Autodesk Inventor part; units mm, degrees
ref_plane "YZ Plane" through (0, 0, 0) normal (1, 0, 0) x (0, 1, 0)
ref_plane "XZ Plane" through (0, 0, 0) normal (0, 1, 0) x (-1, 0, 0)
ref_plane "XY Plane" through (0, 0, 0) normal (0, 0, 1) x (1, 0, 0)
sketch "Sketch1" plane through (0, 0, 0) normal (0, 1, 0) x (-1, 0, 0)
  line L0 (0, 0) -> (0, -57.15)
  line L1 (0, -57.15) -> (31.75, -57.15)
  line L2 (31.75, -57.15) -> (31.75, -82.55)
  line L3 (31.75, -82.55) -> (-57.15, -82.55)
  line L4 (-57.15, -82.55) -> (-57.15, -57.15)
  line L5 (-57.15, -57.15) -> (-25.4, -57.15)
  line L6 (-25.4, -57.15) -> (-25.4, 0)
  line L7 (-25.4, 0) -> (0, 0)
  dimension "d0" = 88.9
  dimension "d1" = 25.4
  dimension "d2" = 25.4
  dimension "d3" = 31.75
  dimension "d4" = 82.55
extrude "Extrusion1" add sketch "Sketch1" along normal blind 2.286
fillet "Fillet1" radius 3.175 2 edges at (25.4, 1.143, -57.15) (0, 1.143, -57.15)
chamfer "Chamfer1" distance 1.5875 angle 45 6 edges at (0, 1.143, 0) (25.4, 1.143, 0) (57.15, 1.143, -57.15) (57.15, 1.143, -82.55) (-31.75, 1.143, -57.15) (-31.75, 1.143, -82.55)
sketch "Sketch2" plane through (0, 2.286, 0) normal (0, 1, 0) x (1, 0, 0)
  line L0 (55.5625, 82.55) -> (-30.1625, 82.55)
  line L1 (25.4, 1.5875) -> (25.4, 53.975)
  point P0 (0, 0)
  point P1 (12.7, 69.85)
  dimension "d11" = 12.7
  dimension "d12" = 12.7
hole "Hole1" at (12.7, 2.286, -69.85) direction (0, -1, 0) diameter 4.1402 end through all
pattern_linear "Rectangular Pattern1" count 6 spacing 12.7 along (0, 0, 1) of "Hole1"
pattern_linear "Rectangular Pattern2" count 7 spacing 12.7 along (-1, 0, 0) of "Hole1" first direction both ways yes
properties part number "T Gusset"
Source: CAD feature listing. Evaluate the final solid. Frame: model axes, mm. A direction names the side the tool comes from. Coordinates: 2 decimals unless noted, no trailing zeros. Loops run counter-clockwise (first coordinate to the right, second up) from the corner with the lowest first, then second, coordinate; pieces in that order, holes last. Notation, with made-up numbers: (44.5, 31.5) - (102.5, 31.5) arc R24 ccw to (102.5, 52.5) - close; hole circle Ø1 at (-39, 68). An arc over 180 degrees is marked (long way). Return JSON: item names as keys, results as strings.
Q1. Material intervals for line 1 along Z through (x, y) = (-12.5, 0.7); line 2 along X through (y, z) = (1.3, -9); line 3 along X through (y, z) = (0.7, -44.45), sorted ascending.
Results:
{"line 1": "-82.55 to -71.91, -67.79 to -57.15", "line 2": "0 to 25.4", "line 3": "0 to 10.63, 14.77 to 25.4"}
Q2. Section B-B, the plane x = -25.4. Return loops of the section in (y, z), plus the area to 3 significant figures.
Results:
{"outline": "(0, -82.55) - (2.29, -82.55) - (2.29, -71.92) - (0, -71.92) - close; (0, -67.78) - (2.29, -67.78) - (2.29, -57.15) - (0, -57.15) - close", "area": "48.6 mm2"}
Q3. Mould query, pull axis Z, two halves, no side actions, for faces 3 (the cylindrical face through (38.01, 1.13, -71.92)), 4 (the flat face through (57.15, 1, -70)), 5 (the flat face through (13, 1, 0)). Classes: released by +Z, released by -Z, zero draft, split by the parting line, or undercut.
Results:
{"face 3": "undercut", "face 4": "zero draft", "face 5": "released by +Z"}
Q4. Contact query for flat-ended pins moving along their axis: P1, Ø1.1, axis at y = 1, z = -28, coming from the +X side; P2, Ø3.5, axis at x = 0, z = -69.85, coming from the -Y side; P3, Ø0.7, axis at x = 46.5, y = 1, coming from the +Z side. Output: stop coordinate, or through.
Results:
{"P1": "x = 25.4", "P2": "through", "P3": "z = -57.15"}
Q5. Section C-C, the plane x = 12.7. Return loops of the section in (y, z), plus the area to 3 significant figures.
Results:
{"outline": "(0, -82.55) - (2.29, -82.55) - (2.29, -71.92) - (0, -71.92) - close; (0, -67.78) - (2.29, -67.78) - (2.29, -59.22) - (0, -59.22) - close; (0, -55.08) - (2.29, -55.08) - (2.29, -46.52) - (0, -46.52) - close; (0, -42.38) - (2.29, -42.38) - (2.29, -33.82) - (0, -33.82) - close; (0, -29.68) - (2.29, -29.68) - (2.29, -21.12) - (0, -21.12) - close; (0, -16.98) - (2.29, -16.98) - (2.29, -8.42) - (0, -8.42) - close; (0, -4.28) - (2.29, -4.28) - (2.29, 0) - (0, 0) - close", "area": "132 mm2"}
Q6. Section A-A, the plane z = -69.85. Give the number of separate pieces and of enclosed holes in the cut face, plus the area to 3 significant figures.
Results:
{"separate pieces": "8", "enclosed holes": "0", "area": "137 mm2"}
Q7. Access query for faces 1 (the cylindrical face through (-12.79, 1.13, -71.92)), 2 (the flat face through (25.4, 1, -28)). Directions: +Z, -Z, +X, -X, +Y, -Y. A direction counts if a zero-diameter tool reaches every point of the face in a straight line with its end or side. Return the directions, or none.
Results:
{"face 1": "+Y, -Y", "face 2": "+Z, +X, +Y, -Y"}
